For this review, take the finished solid that the model builds, in its own axes (mm). Face numbers are marked on the shaded views. A direction names the side the tool comes from. Coordinates: 2 decimals unless noted, no trailing zeros. Write each loop counter-clockwise with the first axis right and the second up, starting at its lowest first coordinate (ties: lowest second). Pieces come first, ordered by that corner, then holes. Notation, with made-up numbers: M 31.5,-18.75 L 53.5,-18.75 A14 ccw 53.5,5.25 Z; hole C -37,81 d3. An arc over 180 degrees is marked long. Return JSON: item names as keys, results as strings.
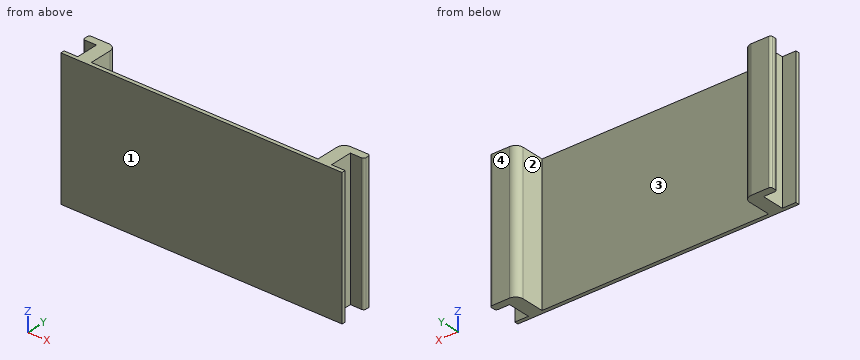
```python
from build123d import *

# Parameters (mm, degrees)
BOSS_EXTRUDE1_DEPTH = 18
FILLET1_R           = 1
FILLET2_R           = 0.3


with BuildPart() as part:
    # Sketch1 → Boss-Extrude1 (new body)
    with BuildSketch(Plane.XY):
        Polygon((-15, 0), (-15, 4), (-18.6, 4), (-18.6, 3), (-16.8, 3), (-16.8, 0), (-18.6, 0), (-18.6, -0.5), (18.6, -0.5), (18.6, 0), (16.8, 0), (16.8, 3), (18.6, 3), (18.6, 4), (15, 4), (15, 0), align=None)
    extrude(amount=BOSS_EXTRUDE1_DEPTH)

    # Fillet1
    fillet1_edges = [part.edges().sort_by_distance(p)[0] for p in [
        (-15, 4, 9),
        (15, 4, 9),
    ]]
    fillet(fillet1_edges, radius=FILLET1_R)

    # Fillet2
    fillet2_edges = [part.edges().sort_by_distance(p)[0] for p in [
        (-18.6, 3, 9),
        (-18.6, 4, 9),
        (18.6, 4, 9),
        (18.6, 3, 9),
    ]]
    fillet(fillet2_edges, radius=FILLET2_R)


solid = part.part
```
1. We need section C-C (x = 7.5). State the section outline as (y, z) points, plus the area to 3 significant figures.
Checks:
{"outline": "M -0.5,0 L 0,0 L 0,18 L -0.5,18 Z", "area": "9.00 mm2"}
2. For the marked faces 1 and 2, list the 3-axis set-ups (+Z, -Z, +X, -X, +Y, -Y) from which the entire face can be reached by the end or side of a thin tool; tool diameter is ignored.
Checks:
{"face 1": "+Z, -Z, +X, -X, -Y", "face 2": "+Z, -Z, +Y"}
3. We need section A-A (y = 1.3). State the section outline as (x, z) points, plus the area to 3 significant figures.
Checks:
{"outline": "M -16.8,0 L -15,0 L -15,18 L -16.8,18 Z; M 15,0 L 16.8,0 L 16.8,18 L 15,18 Z", "area": "64.8 mm2"}
4. Draft analysis for pull direction X (two halves, no side actions). For the marked faces 3 and 4, state which applies: +X half, -X half, draft (parallel to the pull), parting line (faces both ways), or undercut.
Checks:
{"face 3": "undercut", "face 4": "draft"}
5. Clearance check with flat-ended pins moving along their axes: pin 1 Ø9 at (x, z) = (-6.5, 10) entering from +Y; pin 2 Ø0.9 at (y, z) = (1.5, 5) entering from +X; pin 3 Ø0.9 at (y, z) = (1, 12) entering from -X. State where each tip first meets the part, or that it passes through.
Checks:
{"pin 1": "y = 0", "pin 2": "x = 16.8", "pin 3": "x = -16.8"}
6. We need section B-B (z = 5.75). State the section outline as (x, y) points, plus the area to 3 significant figures.
Checks:
{"outline": "M -18.6,-0.5 L 18.6,-0.5 L 18.6,0 L 16.8,0 L 16.8,3 L 18.3,3 A0.3 ccw 18.6,3.3 L 18.6,3.7 A0.3 ccw 18.3,4 L 16,4 A1 ccw 15,3 L 15,0 L -15,0 L -15,3 A1 ccw -16,4 L -18.3,4 A0.3 ccw -18.6,3.7 L -18.6,3.3 A0.3 ccw -18.3,3 L -16.8,3 L -16.8,0 L -18.6,0 Z", "area": "36.1 mm2"}
7. Wall thickness on L1, parallel to X at y = 2, z = 3.5; L2, parallel to Y at x = 10, z = 4.25; L3, parallel to X at y = 3.15, z = 12: over which ranges is each line inside the solid? List them lowest first. Write a range as from..to.
Checks:
{"L1": "-16.8..-15, 15..16.8", "L2": "-0.5..0", "L3": "-18.56..-15.01, 15.01..18.56"}
